Geometry: final body of the model. Coordinates: model frame, mm. Give positions to 0.01 mm unless a question says otherwise; leave off trailing zeros. Order: outer loops, then holes, each group sorted by start corner. A loop starts at its lowest first (then second) coordinate and runs counter-clockwise, first axis right, second up. Notation, with made-up numbers: (-30.75, -39) - (-8.75, -39) arc R16 ccw to (-8.75, -12) - close; hole circle Ø5 at (-40, 70). An arc over 180 degrees is marked (long way). Put each result on its own line as item: value. Start each with the question number.
1. First-contact query: P1, Ø6, axis at x = 4.5, y = 11.5, coming from the -Z side. Flat tip, straight axial feed; report the tip coordinate or a pass-through.
2. Ray query, line 1 along Z through (x, y) = (11, 1). Return the intervals inside material, ascending. Write a range as from..to.
3. Section A-A on y = -12.5. Return the cut outline in (x, z), plus the area to 3 significant figures.
4. Section B-B on x = 12.5. Return the cut outline in (y, z).
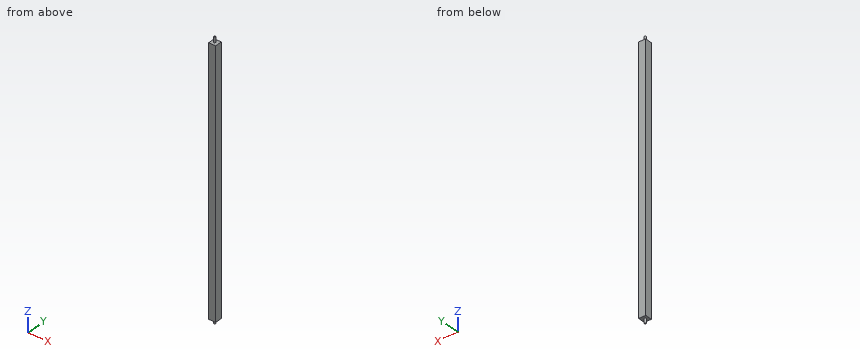
from build123d import *

# Parameters (mm, degrees)
F0_W     = 40
F0_H     = 40
F1_DEPTH = 1490
F2_R     = 4.9
F3_DEPTH = 30
F4_R     = 4.9
F5_DEPTH = 25


with BuildPart() as f1:
    # F0 (on Top) → F1 (new body)
    with BuildSketch(Plane.XY):
        with Locations((1.785715, 0)):
            Rectangle(F0_W, F0_H)
    extrude(amount=F1_DEPTH)

    # F2 (on face) → F3 (join)
    with BuildSketch(Plane.XY.offset(1490)):
        Circle(F2_R)
    extrude(amount=F3_DEPTH)

    # F4 (on face) → F5 (join)
    with BuildSketch(Plane(origin=(0, 0, 0), x_dir=(1, 0, 0), z_dir=(0, 0, -1))):
        Circle(F4_R)
    extrude(amount=F5_DEPTH)


solid = f1.part
Resolved:
1. P1: z = 0
2. line 1: 0..1490
3. outline: (-18.21, 0) - (21.79, 0) - (21.79, 1490) - (-18.21, 1490) - close
3. area: 59,600 mm^2
4. outline: (-20, 0) - (20, 0) - (20, 1490) - (-20, 1490) - close
